The model under review builds one solid part; all positions refer to its coordinate system, in mm. Face numbers are marked on the shaded views. A direction names the side the tool comes from. Coordinates: 2 decimals unless noted, no trailing zeros. Loops run counter-clockwise (first coordinate to the right, second up) from the corner with the lowest first, then second, coordinate; pieces in that order, holes last. Notation, with made-up numbers: M 4,-13 L 38,-13 A30 ccw 38,16 Z; hole C -13.75,-34.5 d1. An arc over 180 degrees is marked long. Write item = value, one per line. Start each with the question number.
Q1. For the marked faces 1, 2 and 3, list the 3-axis set-ups (+Z, -Z, +X, -X, +Y, -Y) from which the entire face can be reached by the end or side of a thin tool; tool diameter is ignored.
Q2. We need section A-A on x = -27.95. Give the boundary of the cut face in (y, z), and give its area (3 significant figures).
Q3. Mouldability with a two-part tool opening along Z and no side actions: class the marked faces 4, 5, 6 and 7 as released by +Z, released by -Z, zero draft, split by the parting line, or undercut.
Q4. Clearance check with flat-ended pins moving along their axes: pin 1 Ø4 at (x, z) = (-2, -24.5) entering from -Y; pin 2 Ø3.5 at (x, z) = (-27.95, -30) entering from +Y; pin 3 Ø6.5 at (y, z) = (35, -5.75) entering from -X. State where each tip first meets the part, or that it passes through.
Q5. We need section C-C on y = 31. Give the boundary of the cut face in (x, z).
Q6. We need section B-B on z = -37. Give the boundary of the cut face in (x, y), and give its area (3 significant figures).
Q7. We need section D-D on z = -5.75. Give the boundary of the cut face in (x, y).
Q8. Wall thickness on probe 1 along Y at (x, z) = (-1.8, -54.25); probe 2 along Y at (x, z) = (-2, -5); probe 3 along Y at (x, z) = (-13.5, -37): over which ranges is each line inside the solid? List them lowest first.
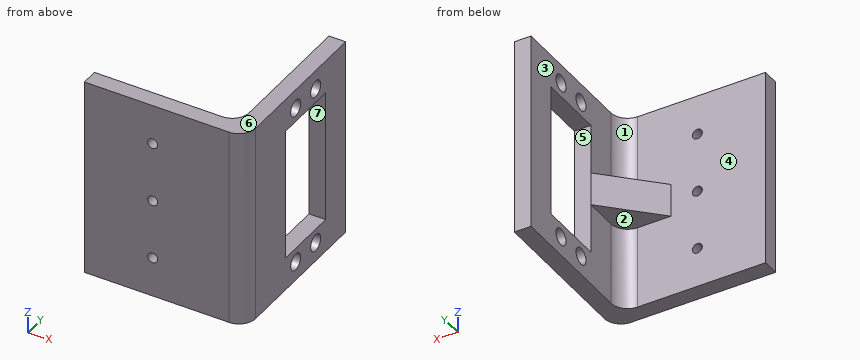
from build123d import *

# Parameters (mm, degrees)
BOSS_EXTRUDE1_DEPTH = 60
SKETCH2_R           = 2.5
SKETCH2_W           = 40
SKETCH2_H           = 20
CUT_EXTRUDE1_DEPTH  = 10
SKETCH3_R           = 1.5
CUT_EXTRUDE2_DEPTH  = 10
RIB1_REACH          = 77.812
SKETCH4_WALL_W      = 174.836453632
SKETCH4_WALL_H      = 10
FILLET1_R           = 5


with BuildPart() as part:
    # Sketch1 → Boss-Extrude1 (new body)
    with BuildSketch(Plane.XY):
        Polygon((0, 0), (0, 50), (-5, 50), (-5, 5), (-48.45, 5), (-48.45, 0), align=None)
    extrude(amount=-BOSS_EXTRUDE1_DEPTH)

    # Sketch2 → Cut-Extrude1 (cut)
    with BuildSketch(Plane(origin=(0, 0, 0), x_dir=(0, 0, -1), z_dir=(1, 0, 0))):
        with Locations((54.25, 35)):
            Circle(SKETCH2_R)
        with Locations(Location((54.25, 25, 0), (0, 0, 270))):
            Circle(SKETCH2_R)
        with Locations((5.75, 25)):
            Circle(SKETCH2_R)
        with Locations(Location((5.75, 35, 0), (0, 0, 270))):
            Circle(SKETCH2_R)
        with Locations((30, 30)):
            Rectangle(SKETCH2_W, SKETCH2_H)
    extrude(amount=-CUT_EXTRUDE1_DEPTH, mode=Mode.SUBTRACT)

    # Sketch3 → Cut-Extrude2 (cut)
    with BuildSketch(Plane.XZ):
        with Locations(Location((-27.95, -30, 0), (0, 0, 270))):
            Circle(SKETCH3_R)
        with Locations(Location((-27.95, -12, 0), (0, 0, 270))):
            Circle(SKETCH3_R)
        with Locations(Location((-27.95, -48, 0), (0, 0, 270))):
            Circle(SKETCH3_R)
    extrude(amount=-CUT_EXTRUDE2_DEPTH, mode=Mode.SUBTRACT)

    # Sketch4 wall → Rib1 (add, up to next)
    with BuildSketch(Plane(origin=(-12.5, 12.5, -30), x_dir=(-0.707106781187, -0.707106781187, 0), z_dir=(0.707106781187, -0.707106781187, 0)), mode=Mode.PRIVATE) as rib1_sk1:
        Rectangle(SKETCH4_WALL_W, SKETCH4_WALL_H)
    rib1_tool1 = extrude(rib1_sk1.sketch, amount=RIB1_REACH, mode=Mode.PRIVATE) - part.part
    add(rib1_tool1.solids().sort_by_distance((-12.5, 12.5, -30))[0])

    # Fillet1
    fillet1_edges = [part.edges().sort_by_distance(p)[0] for p in [
        (-5, 5, -47.5),
        (0, 0, -30),
        (-5, 5, -12.5),
    ]]
    fillet(fillet1_edges, radius=FILLET1_R)


solid = part.part
Returned:
q1.face_1 = +Z, -X, +Y
q1.face_2 = -Z, -X, +Y
q1.face_3 = -X, +Y
q2.outline = M 0,-60 L 5,-60 L 5,-49.5 L 0,-49.5 Z; M 0,-46.5 L 5,-46.5 L 5,-31.5 L 0,-31.5 Z; M 0,-28.5 L 5,-28.5 L 5,-13.5 L 0,-13.5 Z; M 0,-10.5 L 5,-10.5 L 5,0 L 0,0 Z
q2.area = 255 mm^2
q3.face_4 = zero draft
q3.face_5 = undercut
q3.face_6 = released by +Z
q3.face_7 = undercut
q4.pin_1 = 0.1
q4.pin_2 = 5
q4.pin_3 = -5
q5.outline = M -5,-60 L 0,-60 L 0,-50 L -5,-50 Z; M -5,-10 L 0,-10 L 0,0 L -5,0 Z
q6.outline = M -48.45,0 L -5,0 A5 ccw 0,5 L 0,20 L -5,20 L -5,10 A5 cw -10,5 L -48.45,5 Z; M -5,40 L 0,40 L 0,50 L -5,50 Z
q6.area = 367 mm^2
q7.outline = M -48.45,0 L -5,0 A5 ccw 0,5 L 0,22.5 L -5,22.5 L -5,10 A5 cw -10,5 L -48.45,5 Z; M -5,27.5 L 0,27.5 L 0,32.5 L -5,32.5 Z; M -5,37.5 L 0,37.5 L 0,50 L -5,50 Z
q8.probe_1 = 1.16 to 22.5, 27.5 to 32.5, 37.5 to 50
q8.probe_2 = 1 to 22.62, 27.38 to 32.62, 37.38 to 50
q8.probe_3 = 0 to 5
